Read the model definition and answer for the solid it produces. Units are mm, in the model's axes. Round coordinates to 2 decimals unless told otherwise and drop trailing zeros. Write each loop counter-clockwise with the first axis right and the second up, starting at its lowest first coordinate (ties: lowest second). Pieces come first, ordered by that corner, then holes. Notation, with made-up numbers: (55, 0.5) -> (103, 0.5) arc R21 cw to (103, 20.5) -> close; hole circle Ø1 at (31.25, -12). An arc over 180 degrees is marked (long way). Return JSON: item names as keys, results as strings.
from build123d import *

# Parameters (mm, degrees)
SKETCH_W      = 30
SKETCH_H      = 30
SKETCH_R      = 4
SKETCH_R_2    = 1.55
EXTRUDE_DEPTH = 2
FILLET_R      = 4


with BuildPart() as part:
    # Sketch → Extrude (new body)
    with BuildSketch(Plane.XY):
        Rectangle(SKETCH_W, SKETCH_H)
        Circle(SKETCH_R, mode=Mode.SUBTRACT)
        with Locations((-11, 11)):
            Circle(SKETCH_R_2, mode=Mode.SUBTRACT)
        with Locations((-11, -11)):
            Circle(SKETCH_R_2, mode=Mode.SUBTRACT)
        with Locations((11, -11)):
            Circle(SKETCH_R_2, mode=Mode.SUBTRACT)
        with Locations((11, 11)):
            Circle(SKETCH_R_2, mode=Mode.SUBTRACT)
    extrude(amount=EXTRUDE_DEPTH)

    # Fillet
    fillet_edges = [part.edges().sort_by_distance(p)[0] for p in [
        (-15, -15, 1),
        (15, -15, 1),
        (15, 15, 1),
        (-15, 15, 1),
    ]]
    fillet(fillet_edges, radius=FILLET_R)


solid = part.part
Item 1: Section B-B (x = -3) is taken. Give the vertices of the cut face in (y, z), then the cut area to 3 significant figures.
Worked answers:
{"outline": "(-15, 0) -> (-2.65, 0) -> (-2.65, 2) -> (-15, 2) -> close; (2.65, 0) -> (15, 0) -> (15, 2) -> (2.65, 2) -> close", "area": "49.4 mm2"}
Item 2: For a pull along X with two mould halves and no side action, classify faces 1 (the flat face through (3, -3, 0)), 2 (the cylindrical face through (13.797, 13.859, 1.014)), 3 (the cylindrical face through (9.77, -11.94, 0.99)) as released by +X, released by -X, zero draft, split by the parting line, or undercut.
Worked answers:
{"face 1": "zero draft", "face 2": "released by +X", "face 3": "undercut"}
Item 3: A flat-ended cylindrical pin translates along its axis: pin 1 (6.5 mm diameter, centred on x = 0, y = 0, fed in from +Z). Find the tip coordinate at first contact, or state that the pin passes through.
Worked answers:
{"pin 1": "passes through"}
Item 4: Section C-C (z = 0.6) is taken. Give the vertices of the cut face in (x, y), then the cut area to 3 significant figures.
Worked answers:
{"outline": "(-15, -11) arc R4 ccw to (-11, -15) -> (11, -15) arc R4 ccw to (15, -11) -> (15, 11) arc R4 ccw to (11, 15) -> (-11, 15) arc R4 ccw to (-15, 11) -> close; hole circle Ø3.1 at (-11, -11); hole circle Ø3.1 at (-11, 11); hole circle Ø8 at (0, 0); hole circle Ø3.1 at (11, -11); hole circle Ø3.1 at (11, 11)", "area": "806 mm2"}
Item 5: Section A-A (y = 0) is taken. Give the vertices of the cut face in (x, z), then the cut area to 3 significant figures.
Worked answers:
{"outline": "(-15, 0) -> (-4, 0) -> (-4, 2) -> (-15, 2) -> close; (4, 0) -> (15, 0) -> (15, 2) -> (4, 2) -> close", "area": "44.0 mm2"}
Item 6: Straight lines are drawn through the part: L1, parallel to Y at x = -11, z = 1.1; L2, parallel to Y at x = 0, z = 1; L3, parallel to X at y = 11.75, z = 0.5. For each, find the intervals that lie inside material, in ascending order. Write a range as [from, to].
Worked answers:
{"L1": "y = [-15, -12.55], [-9.45, 9.45], [12.55, 15]", "L2": "y = [-15, -4], [4, 15]", "L3": "x = [-14.93, -12.36], [-9.64, 9.64], [12.36, 14.93]"}
